Answer from the drawing. Dimensions are ordinates in mm from the lowest x, y and z of the part. A direction names the side the tool comes from. Give positions to 0.01 mm unless a question says otherwise; leave off trailing zeros. Write each loop counter-clockwise with the first axis right and the second up, starting at its lowest first coordinate (ties: lowest second). Pieces come first, ordered by that corner, then holes. Notation, with made-up numbers: (19, 12.5) - (43, 12.5) arc R19 cw to (43, 43.5) - close; hole circle Ø4 at (31.5, 38.25). An arc over 180 degrees is marked (long way). Answer as a JSON object with one key per item and string values. Group by question number.
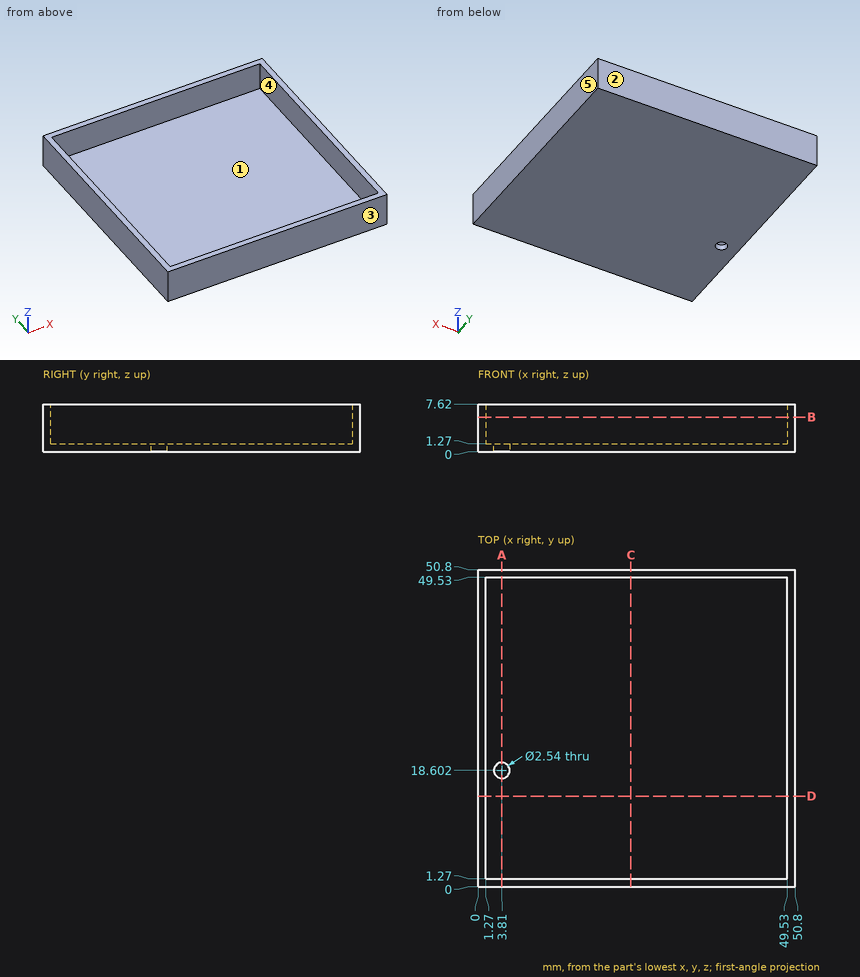
1) For a pull along Y with two mould halves and no side action, classify the marked faces 1, 2 and 3 as released by +Y, released by -Y, zero draft, split by the parting line, or undercut.
2) Find section A-A, the plane x = 3.81. Write down the section's boundary in (y, z).
3) Find section C-C, the plane x = 24.5. Write down the section's boundary in (y, z).
4) Which of the six approach directions +Z, -Z, +X, -X, +Y, -Y give full straight-line access (tool end or side, diameter ignored) to the marked faces 4 and 5?
5) Find section B-B, the plane z = 5.5. Write down the section's boundary in (x, y).
6) Find the intervals of material crossed by line 1 (X direction, y = 26, z = 2.75); line 2 (Y direction, x = 3.81, z = 0.3), in increasing order. Write a range as [from, to].
Values follow:
{
 "1": {"face 1": "undercut", "face 2": "released by +Y", "face 3": "released by -Y"},
 "2": {"outline": "(0, 0) - (17.33, 0) - (17.33, 1.27) - (1.27, 1.27) - (1.27, 7.62) - (0, 7.62) - close; (19.87, 0) - (50.8, 0) - (50.8, 7.62) - (49.53, 7.62) - (49.53, 1.27) - (19.87, 1.27) - close"},
 "3": {"outline": "(0, 0) - (50.8, 0) - (50.8, 7.62) - (49.53, 7.62) - (49.53, 1.27) - (1.27, 1.27) - (1.27, 7.62) - (0, 7.62) - close"},
 "4": {"face 4": "+Z", "face 5": "+Z, -Z, +X, +Y, -Y"},
 "5": {"outline": "(0, 0) - (50.8, 0) - (50.8, 50.8) - (0, 50.8) - close; hole (1.27, 1.27) - (49.53, 1.27) - (49.53, 49.53) - (1.27, 49.53) - close"},
 "6": {"line 1": "x = [0, 1.27], [49.53, 50.8]", "line 2": "y = [0, 17.33], [19.87, 50.8]"}
}
